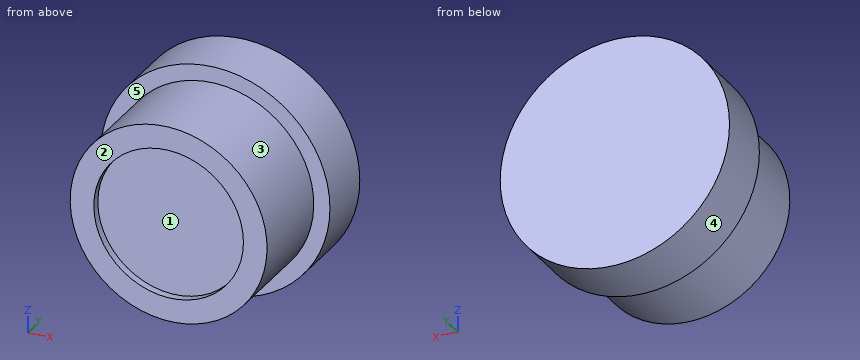
```python
from build123d import *


with BuildPart() as f2:
    # F0 (on Right) → F2 (revolve)
    with BuildSketch(Plane.YZ):
        Polygon((5.0038, 47.498), (5.0038, 0), (57.9374, 0), (57.9374, 62.4967), (0, 62.4967), (0, 47.498), align=None)
        Polygon((57.9374, 62.4967), (57.9374, 0), (94.996, 0), (94.996, 72.7837), (57.9374, 72.7837), align=None)
    revolve(axis=Axis((0, 35.516532, 0), (0, 1, 0)))


solid = f2.part
```
Geometry check sheet. Reference: the model listing, model coordinates, mm. Face numbers are marked on the shaded views. A direction names the side the tool comes from. Give positions to 0.01 mm unless a question says otherwise; leave off trailing zeros. Order: outer loops, then holes, each group sorted by start corner. A loop starts at its lowest first (then second) coordinate and runs counter-clockwise, first axis right, second up. Notation, with made-up numbers: (48, 63) -> (66, 63) arc R24 ccw to (66, 77) -> close; hole circle Ø8 at (54, 42). An arc over 180 degrees is marked (long way). Write each question's results on one line, items separated by ' | '. Start each with the question number.
(1) Sectioned sample at A-A (x = 0). Enter the section's corners in (y, z).
(2) Sectioned sample at D-D (x = -50). Enter the section's corners in (y, z), plus the area to 3 significant figures.
(3) Sectioned sample at B-B (z = 0). Enter the section's corners in (x, y).
(4) Sectioned sample at C-C (y = 84). Enter the section's corners in (x, z), plus the area to 3 significant figures.
(5) Access from +Z, -Z, +X, -X, +Y, -Y to the whole of each face (thin tool, end or side, straight path). Record for the marked faces 4 and 5.
(6) Mould release check, pull along X, two halves, no side actions. Record for the marked faces 1, 2 and 3: pulls with the +X half, pulls with the -X half, needs draft (parallel to the pull), parting line crosses it, or undercut.
(7) Gauge pin test, flat ends, axial feed: P1, Ø12, axis at x = -23, y = 19, coming from the -Z side; P2, Ø5, axis at x = -57.5, z = 31, coming from the -Y side; P3, Ø5, axis at x = -5, y = 26.5, coming from the +Z side. Record the tip position at first contact, or that the pin passes through.
(8) Scan lines: line 1 (X direction, y = 1, z = 0); line 2 (Y direction, x = -25, z = 17.5); line 3 (Y direction, x = -14.5, z = 64). Record each from-to range of solid material in increasing order.
Answer below:
1) outline: (0, -62.5) -> (57.94, -62.5) -> (57.94, -72.78) -> (95, -72.78) -> (95, 72.78) -> (57.94, 72.78) -> (57.94, 62.5) -> (0, 62.5) -> (0, 47.5) -> (5, 47.5) -> (5, -47.5) -> (0, -47.5) -> close
2) outline: (0, -37.49) -> (57.94, -37.49) -> (57.94, -52.89) -> (95, -52.89) -> (95, 52.89) -> (57.94, 52.89) -> (57.94, 37.49) -> (0, 37.49) -> close | area: 8,260 mm2
3) outline: (-72.78, 57.94) -> (-62.5, 57.94) -> (-62.5, 0) -> (-47.5, 0) -> (-47.5, 5) -> (47.5, 5) -> (47.5, 0) -> (62.5, 0) -> (62.5, 57.94) -> (72.78, 57.94) -> (72.78, 95) -> (-72.78, 95) -> close
4) outline: circle Ø145.57 at (0, 0) | area: 16,600 mm2
5) face 4: +Y, -Y | face 5: -Y
6) face 1: undercut | face 2: needs draft | face 3: parting line crosses it
7) P1: z = -60.14 | P2: y = 57.94 | P3: z = 62.45
8) line 1: -62.5 to -47.5, 47.5 to 62.5 | line 2: 5 to 95 | line 3: 57.94 to 95
